from build123d import *

# Parameters (mm, degrees)
BOSS_EXTRUDE1_DEPTH = 10
SKETCH2_R           = 1.75
CUT_EXTRUDE1_DEPTH  = 35
DRAFT1_ANGLE        = 2
BOSS_EXTRUDE2_DEPTH = 2.5
SKETCH6_W           = 26
SKETCH6_H           = 76
CUT_EXTRUDE4_DEPTH  = 2
SKETCH7_W           = 5
SKETCH7_H           = 7
CUT_EXTRUDE5_DEPTH  = 1
CUT_EXTRUDE6_DEPTH  = 5
SKETCH9_W           = 21
SKETCH9_H           = 55
CUT_EXTRUDE7_DEPTH  = 2


with BuildPart() as part:
    # Sketch1 → Boss-Extrude1 (new body)
    with BuildSketch(Plane(origin=(0, 0, 0), x_dir=(0, 0, -1), z_dir=(1, 0, 0))):
        Polygon((19.10611554, 15.010195009), (28.614736708, 20.5), (32.149736708, 14.377200395), (32.149736708, 0), (19.10611554, 0), align=None)
    extrude(amount=BOSS_EXTRUDE1_DEPTH)

    # Sketch2 → Cut-Extrude1 (cut)
    with BuildSketch(Plane(origin=(0, 17.515544456, -30.33781292), x_dir=(1, 0, 0), z_dir=(0, 0.5000000000000014, -0.8660254037844378))):
        with Locations(Location((5, 0.053847576, 0), (0, 0, 270))):
            Circle(SKETCH2_R)
    extrude(amount=-CUT_EXTRUDE1_DEPTH, mode=Mode.SUBTRACT)

    # Draft1
    draft1_faces = [part.faces().sort_by_distance(p)[0] for p in [
        (5, 12.426932649, -25.131773882),
    ]]
    draft(draft1_faces, Plane(origin=(10, 20.5, -28.614736708), x_dir=(0, -0.8660254037844377, -0.5000000000000018), z_dir=(0, 0.5000000000000017, -0.8660254037844376)), DRAFT1_ANGLE)

    # Sketch5 → Boss-Extrude2 (add)
    with BuildSketch(Plane.XZ):
        Polygon((11.5, 76), (-20.5, 76), (-20.5, -5), (-6.5, -5), (-6.5, -32.15), (11.5, -32.15), align=None)
    extrude(amount=BOSS_EXTRUDE2_DEPTH)

    # Sketch6 → Cut-Extrude4 (cut)
    with BuildSketch(Plane(origin=(0, 0, 0), x_dir=(1, 0, 0), z_dir=(0, 1, 0))):
        with Locations((-4.5, -35)):
            Rectangle(SKETCH6_W, SKETCH6_H)
    extrude(amount=-CUT_EXTRUDE4_DEPTH, mode=Mode.SUBTRACT)

    # Sketch7 → Cut-Extrude5 (cut)
    with BuildSketch(Plane(origin=(0, -2, 0), x_dir=(1, 0, 0), z_dir=(0, 1, 0))):
        with Locations((4.5, -8.75)):
            Rectangle(SKETCH7_W, SKETCH7_H)
    extrude(amount=-CUT_EXTRUDE5_DEPTH, mode=Mode.SUBTRACT)

    # Sketch8 → Cut-Extrude6 (cut)
    with BuildSketch(Plane(origin=(0, 0, 73), x_dir=(-1, 0, 0), z_dir=(0, 0, -1))):
        with BuildLine():
            Line((-5.5, 0), (10.5, 0))
            ThreePointArc((10.5, 0), (2.5, -2.31142246), (-5.5, 0))
        make_face()
    extrude(amount=-CUT_EXTRUDE6_DEPTH, mode=Mode.SUBTRACT)

    # Sketch9 → Cut-Extrude7 (cut)
    with BuildSketch(Plane(origin=(0, 0, 0), x_dir=(1, 0, 0), z_dir=(0, 1, 0))):
        with Locations((1, -17.5)):
            Rectangle(SKETCH9_W, SKETCH9_H)
    extrude(amount=-CUT_EXTRUDE7_DEPTH, mode=Mode.SUBTRACT)


solid = part.part
Can you work these out from the model? Positions are in its coordinate system, mm. A direction names the side the tool comes from. Coordinates: 2 decimals unless noted, no trailing zeros. Write each loop counter-clockwise with the first axis right and the second up, starting at its lowest first coordinate (ties: lowest second). Pieces come first, ordered by that corner, then holes. Notation, with made-up numbers: (-33.5, -7.75) -> (-16.5, -7.75) arc R18 cw to (-16.5, 23.25) -> close; hole circle Ø8 at (36, 46.25). An arc over 180 degrees is marked (long way). Write each question's results on one line, items separated by ' | '. Start each with the question number.
Item 1: If we section it at A-A, the plane z = 59.5: Write out the boundary of the cut face in (x, y), and give its area (3 significant figures).
Item 2: I'm going to push flat-ended pins straight in: P1, Ø6.5, axis at x = 7.5, z = 63, coming from the +Y side; P2, Ø0.8, axis at y = -1.5, z = -14.5, coming from the -X side; P3, Ø5.5, axis at x = 7, z = -22.5, coming from the +Y side. Where does each tip first touch, or does it pass through?
Item 3: On a 3-axis mill with a long thin cutter (end or side, diameter ignored), from which of +Z, -Z, +X, -X, +Y, -Y can I reach the whole of each face in a straight line? I mean faces 1 (the flat face through (-15, -1, -5)), 2 (the flat face through (-13, -1, 73)), 3 (the flat face through (-9.5, -1, -4)). Say none if no direction works.
Item 4: If we section it at C-C, the plane y = 1: Write out the boundary of the cut face in (x, z).
Item 5: If we section it at B-B, the plane x = -16: Write out the boundary of the cut face in (y, z).
Item 6: Thinking about a two-plate mould opening in Z: for faces 4 (the flat face through (5, 7, -19.106)), 5 (the flat face through (10, -1, 45)), 6 (the flat face through (-20.5, -1, 36)), which applies, released by +Z, released by -Z, zero draft, split by the parting line, or undercut?
Item 7: Please list where these lines run through material, in increasing order: probe 1 along X at (y, z) = (-0.25, 70.5); probe 2 along Z at (x, y) = (-15, -0.25); probe 3 along Y at (x, z) = (6, 61.5).
Item 8: If we section it at D-D, the plane z = 44: Write out the boundary of the cut face in (x, y), and give its area (3 significant figures).
Answer block:
1) outline: (-20.5, -2.5) -> (11.5, -2.5) -> (11.5, 0) -> (8.5, 0) -> (8.5, -2) -> (-17.5, -2) -> (-17.5, 0) -> (-20.5, 0) -> close | area: 28.0 mm²
2) P1: y = 0 | P2: x = -6.5 | P3: y = 18.56
3) face 1: -Z, -X, +Y, -Y | face 2: +Y | face 3: -Z, +X, +Y
4) outline: (0, -32.15) -> (10, -32.15) -> (10, -19.11) -> (0, -19.11) -> close
5) outline: (-2.5, -5) -> (0, -5) -> (0, -3) -> (-2, -3) -> (-2, 73) -> (0, 73) -> (0, 76) -> (-2.5, 76) -> close
6) face 4: released by +Z | face 5: undercut | face 6: zero draft
7) probe 1: -20.5 to -17.5, 8.5 to 11.5 | probe 2: -5 to -3, 73 to 76 | probe 3: -2.5 to -2
8) outline: (-20.5, -2.5) -> (11.5, -2.5) -> (11.5, -2) -> (-17.5, -2) -> (-17.5, 0) -> (-20.5, 0) -> close | area: 22.0 mm²
